from build123d import *

# Parameters (mm, degrees)
F0_W      = 100
F0_H      = 155
F1_DEPTH  = 2
F2_W      = 100
F2_H      = 155
F2_W_2    = 96
F2_H_2    = 151
F3_DEPTH  = 45
F4_W      = 41
F4_H      = 81
F5_DEPTH  = 25
F6_R      = 3.5
F7_DEPTH  = 25
F8_W      = 10
F8_H      = 19
F9_DEPTH  = 25
F10_W     = 120
F10_H     = 175
F10_W_2   = 96
F10_H_2   = 151
F11_DEPTH = 10
F12_R     = 2.5
F13_DEPTH = 25
F14_W     = 20
F14_H     = 5
F15_DEPTH = 25
F16_R     = 1.5


with BuildPart() as f1:
    # F0 (on Top) → F1 (new body)
    with BuildSketch(Plane.XY):
        with Locations((3.314801, 2.740827)):
            Rectangle(F0_W, F0_H)
    extrude(amount=F1_DEPTH)

    # F2 (on face) → F3 (join)
    with BuildSketch(Plane.XY.offset(2)):
        with Locations((3.314801, 2.740827)):
            Rectangle(F2_W, F2_H)
        with Locations((3.314801, 2.740827)):
            Rectangle(F2_W_2, F2_H_2, mode=Mode.SUBTRACT)
    extrude(amount=F3_DEPTH)

    # F4 (on face) → F5 (cut)
    with BuildSketch(Plane(origin=(0, 0, 0), x_dir=(1, 0, 0), z_dir=(0, 0, -1))):
        with Locations((12.814801, -2.740827)):
            Rectangle(F4_W, F4_H)
    extrude(amount=-F5_DEPTH, mode=Mode.SUBTRACT)

    # F6 (on face) → F7 (cut)
    with BuildSketch(Plane(origin=(0, 0, 0), x_dir=(1, 0, 0), z_dir=(0, 0, -1))):
        with Locations((-2.685199, 44.759173)):
            Circle(F6_R)
        with Locations((27.314801, 44.759173)):
            Circle(F6_R)
        with Locations((27.314801, -63.240827)):
            Circle(F6_R)
        with Locations((12.314801, -63.240827)):
            Circle(F6_R)
        with Locations((-2.685199, -63.240827)):
            Circle(F6_R)
    extrude(amount=-F7_DEPTH, mode=Mode.SUBTRACT)

    # F8 (on face) → F9 (cut)
    with BuildSketch(Plane(origin=(0, 0, 0), x_dir=(1, 0, 0), z_dir=(0, 0, -1))):
        with Locations((46.314801, 60.259173)):
            Rectangle(F8_W, F8_H)
    extrude(amount=-F9_DEPTH, mode=Mode.SUBTRACT)

    # F10 (on face) → F11 (join)
    with BuildSketch(Plane.XY.offset(47)):
        with Locations((3.314801, 2.740827)):
            Rectangle(F10_W, F10_H)
        with Locations((3.314801, 2.740827)):
            Rectangle(F10_W_2, F10_H_2, mode=Mode.SUBTRACT)
    extrude(amount=-F11_DEPTH)

    # F12 (on face) → F13 (cut)
    with BuildSketch(Plane(origin=(0, 0, 37), x_dir=(1, 0, 0), z_dir=(0, 0, -1))):
        with Locations((-51.685199, -60.240827)):
            Circle(F12_R)
        with Locations((-51.685199, -2.740827)):
            Circle(F12_R)
        with Locations((-51.685199, 54.759173)):
            Circle(F12_R)
        with Locations((58.314801, 54.759173)):
            Circle(F12_R)
        with Locations((58.314801, -2.740827)):
            Circle(F12_R)
        with Locations((58.314801, -60.240827)):
            Circle(F12_R)
    extrude(amount=-F13_DEPTH, mode=Mode.SUBTRACT)

    # F14 (on face) → F15 (cut)
    with BuildSketch(Plane(origin=(0, 80.240827, 0), x_dir=(-1, 0, 0), z_dir=(0, 1, 0))):
        with Locations((-3.314801, 30.98563)):
            Rectangle(F14_W, F14_H)
    extrude(amount=-F15_DEPTH, mode=Mode.SUBTRACT)

    # F16
    f16_edges = [f1.edges().sort_by_distance(p)[0] for p in [
        (-46.685199, 2.740827, 37),
        (3.314801, 80.240827, 37),
        (3.314801, -74.759173, 37),
        (53.314801, 2.740827, 37),
    ]]
    fillet(f16_edges, radius=F16_R)


solid = f1.part
Part model, mm, in its own coordinate system. A direction names the side the tool comes from. Coordinates: 2 decimals unless noted, no trailing zeros. Write each loop counter-clockwise with the first axis right and the second up, starting at its lowest first coordinate (ties: lowest second). Pieces come first, ordered by that corner, then holes. Notation, with made-up numbers: (25, 30) - (49, 30) arc R17 ccw to (49, 49) - close; hole circle Ø2 at (-35.5, 45.5). An arc over 180 degrees is marked (long way). Put each result on its own line as item: value.
1. Probe line 1 along Y through (x, z) = (-27.5, 3); line 2 along Y through (x, z) = (34.5, 39.5); line 3 along X through (y, z) = (-42, 43). List the from-to ranges inside material, lowest first. Write a range as [from, to].
Final values:
line 1: y = [-74.76, -72.76], [78.24, 80.24]
line 2: y = [-84.76, -72.76], [78.24, 90.24]
line 3: x = [-56.69, -44.69], [51.31, 63.31]
2. Band-saw the part on A-A (y = -63). Write the cut outline in (x, z), then the cut area to 3 significant figures.
Final values:
outline: (-56.69, 37) - (-48.19, 37) arc R1.5 cw to (-46.69, 35.5) - (-46.69, 0) - (41.31, 0) - (41.31, 2) - (-44.69, 2) - (-44.69, 47) - (-56.69, 47) - close; (51.31, 0) - (53.31, 0) - (53.31, 35.5) arc R1.5 cw to (54.81, 37) - (63.31, 37) - (63.31, 47) - (51.31, 47) - close
area: 561 mm²
3. 3-axis set-ups, long thin cutter, end or side, ignore diameter. For faces 5 (the flat face through (3, -74.759, 18)), 6 (the flat face through (-44.685, 2, 24)), 7 (the flat face through (3, 80.241, 18)), 8 (the cylindrical face through (-50.341, 58.133, 41.93)), 9 (the flat face through (-50, 10, 37)): which of +Z, -Z, +X, -X, +Y, -Y reach the whole face in a straight line?
Final values:
face 5: -Z, +X, -X, -Y
face 6: +Z
face 7: -Z, +X, -X, +Y
face 8: +Z, -Z
face 9: -Z
4. Band-saw the part on B-B (z = 10). Write the cut outline in (x, y), then the cut area to 3 significant figures.
Final values:
outline: (-46.69, -74.76) - (53.31, -74.76) - (53.31, 80.24) - (-46.69, 80.24) - close; hole (-44.69, -72.76) - (51.31, -72.76) - (51.31, 78.24) - (-44.69, 78.24) - close
area: 1,000 mm²
5. Flat gauge pins, fed straight in: pin 1 Ø9 at (x, y) = (27.31, -44.76) entering from +Z; pin 2 Ø4 at (x, z) = (-43.5, 6) entering from +Y; pin 3 Ø4 at (x, y) = (-43.5, -39) entering from +Z; pin 4 Ø4 at (y, z) = (5.5, 23) entering from -X. Where does each tip first touch, or does it go through?
Final values:
pin 1: stops at z = 2
pin 2: stops at y = 80.24
pin 3: stops at z = 47
pin 4: stops at x = -46.69
6. Two-plate mould, pull along X, no slides. Class faces 1 (the flat face through (2, -84.759, 42)), 2 (the cylindrical face through (-3.14, -48.23, 0.99)), 3 (the flat face through (-46.685, 2, 18)), 4 (the flat face through (3, -72.759, 24)): +X half, -X half, draft (parallel to the pull), parting line (faces both ways), or undercut.
Final values:
face 1: draft
face 2: undercut
face 3: -X half
face 4: undercut
7. Band-saw the part on C-C (x = -26). Write the cut outline in (y, z).
Final values:
outline: (-84.76, 37) - (-76.26, 37) arc R1.5 cw to (-74.76, 35.5) - (-74.76, 0) - (80.24, 0) - (80.24, 35.5) arc R1.5 cw to (81.74, 37) - (90.24, 37) - (90.24, 47) - (78.24, 47) - (78.24, 2) - (-72.76, 2) - (-72.76, 47) - (-84.76, 47) - close
8. Band-saw the part on D-D (z = 39). Write the cut outline in (x, y).
Final values:
outline: (-56.69, -84.76) - (63.31, -84.76) - (63.31, 90.24) - (-56.69, 90.24) - close; hole circle Ø5 at (-51.69, -54.76); hole circle Ø5 at (-51.69, 2.74); hole circle Ø5 at (-51.69, 60.24); hole (-44.69, -72.76) - (51.31, -72.76) - (51.31, 78.24) - (-44.69, 78.24) - close; hole circle Ø5 at (58.31, -54.76); hole circle Ø5 at (58.31, 2.74); hole circle Ø5 at (58.31, 60.24)
